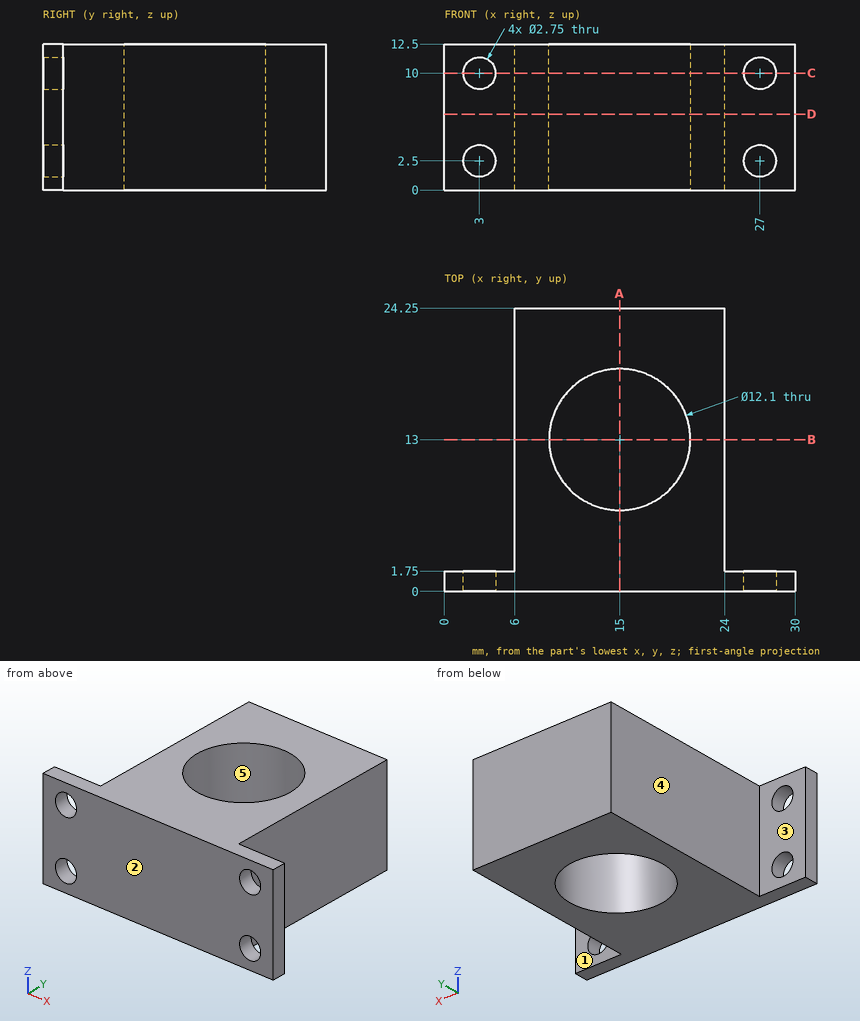
For this review, use the dimensioned drawing (mm, ordinates from the lowest corner) and the shaded views. A direction names the side the tool comes from. Coordinates: 2 decimals unless noted, no trailing zeros. Loops run counter-clockwise (first coordinate to the right, second up) from the corner with the lowest first, then second, coordinate; pieces in that order, holes last.
1. Add section D-D, the plane z = 6.5. Give the boundary of the cut face in (x, y), then the cut area to 3 significant figures.
2. For the marked faces 1 and 2, list the 3-axis set-ups (+Z, -Z, +X, -X, +Y, -Y) from which the entire face can be reached by the end or side of a thin tool; tool diameter is ignored.
3. Add section C-C, the plane z = 10. Give the boundary of the cut face in (x, y) (3 decimals), then the cut area to 3 significant figures.
4. Mouldability with a two-part tool opening along X and no side actions: class the marked faces 3, 4 and 5 as +X half, -X half, draft (parallel to the pull), parting line (faces both ways), or undercut.
5. Add section B-B, the plane y = 13. Give the boundary of the cut face in (x, z).
6. Add section A-A, the plane x = 15. Give the boundary of the cut face in (y, z), then the cut area to 3 significant figures.
7. For line 1 (X direction, y = 0.95, z = 10) (3 decimals); line 2 (Z direction, x = 3, y = 0.95) (3 decimals); line 3 (X direction, y = 6, z = 11.25), list the stretches that pass through material, from the lowest coordinate up.
8. Insertion check: P1, Ø5, axis at y = 5, z = 10.5, coming from the -X side; P2, Ø2.5, axis at x = 27, z = 10, coming from the -Y side; P3, Ø1.5, axis at y = 15.5, z = 6.5, coming from the +X side; P4, Ø3, axis at x = 3, z = 10, coming from the +Y side. Each pin has a flat end and moves straight along its axis. Give the tip position at first contact, or say it passes through.
Result:
1. outline: (0, 0) - (30, 0) - (30, 1.75) - (24, 1.75) - (24, 24.25) - (6, 24.25) - (6, 1.75) - (0, 1.75) - close; hole circle Ø12.1 at (15, 13)
1. area: 343 mm2
2. face 1: +Z, -Z, +X, +Y
2. face 2: +Z, -Z, +X, -X, -Y
3. outline: (0, 0) - (1.625, 0) - (1.625, 1.75) - (0, 1.75) - close; (4.375, 0) - (25.625, 0) - (25.625, 1.75) - (24, 1.75) - (24, 24.25) - (6, 24.25) - (6, 1.75) - (4.375, 1.75) - close; (28.375, 0) - (30, 0) - (30, 1.75) - (28.375, 1.75) - close; hole circle Ø12.1 at (15, 13)
3. area: 333 mm2
4. face 3: draft
4. face 4: -X half
4. face 5: undercut
5. outline: (6, 0) - (8.95, 0) - (8.95, 12.5) - (6, 12.5) - close; (21.05, 0) - (24, 0) - (24, 12.5) - (21.05, 12.5) - close
6. outline: (0, 0) - (6.95, 0) - (6.95, 12.5) - (0, 12.5) - close; (19.05, 0) - (24.25, 0) - (24.25, 12.5) - (19.05, 12.5) - close
6. area: 152 mm2
7. line 1: x = 0 to 1.625, 4.375 to 25.625, 28.375 to 30
7. line 2: z = 0 to 1.125, 3.875 to 8.625, 11.375 to 12.5
7. line 3: x = 6 to 24
8. P1: stops at x = 6
8. P2: passes through
8. P3: stops at x = 24
8. P4: stops at y = 1.75
